The listing builds one solid part. Answer for the finished solid, in the listing's coordinates (mm). Coordinates: 2 decimals unless noted, no trailing zeros. Answer in a Markdown table with one row per item. Add a question column.
```python
from build123d import *

# Parameters (mm, degrees)
BOSS_EXTRUDE1_DEPTH    = 3.175
SKETCH2_R              = 17.4625
CUT_EXTRUDE1_DEPTH     = 435.789559011
F_10_CLEARANCE_HOLE1_D = 5.1054
SKETCH4_R              = 2.794
CUT_EXTRUDE2_DEPTH     = 435.789559011
SKETCH7_R              = 3.048
CUT_EXTRUDE3_DEPTH     = 435.789559011
SKETCH8_R              = 3
CUT_EXTRUDE4_DEPTH     = 435.789559011


with BuildPart() as part:
    # Sketch1 → Boss-Extrude1 (new body)
    with BuildSketch(Plane.XY):
        with BuildLine():
            Line((0, 0), (406.4, 0))
            ThreePointArc((406.4, 0), (431.8, 25.4), (406.4, 50.8))
            Line((406.4, 50.8), (0, 50.8))
            ThreePointArc((0, 50.8), (-25.4, 25.4), (0, 0))
        make_face()
    extrude(amount=BOSS_EXTRUDE1_DEPTH)

    # Sketch2 → Cut-Extrude1 (cut, through all)
    with BuildSketch(Plane.XY.offset(3.175)):
        with Locations((0, 25.4)):
            Circle(SKETCH2_R)
        with Locations((406.4, 25.4)):
            Circle(SKETCH2_R)
    extrude(amount=-CUT_EXTRUDE1_DEPTH, mode=Mode.SUBTRACT)

    # #10 Clearance Hole1 (through all)
    with Locations(Plane(origin=(18.257547563, 35.941, 3.175), x_dir=(1, 0, 0), z_dir=(0, 0, 1))):
        with Locations((0, 0), (0, -21.082), (-18.257547563, -31.623), (-36.515095126, -21.082), (-36.515095126, 0), (-18.257547563, 10.541)):
            Hole(F_10_CLEARANCE_HOLE1_D / 2)

    # Sketch4 → Cut-Extrude2 (cut, through all)
    with BuildSketch(Plane.XY.offset(3.175)):
        with Locations((101.6, 25.4)):
            Circle(SKETCH4_R)
        with Locations((127, 25.4)):
            Circle(SKETCH4_R)
        with Locations((184.272931293, 25.4)):
            Circle(SKETCH4_R)
        with Locations((209.672931293, 25.4)):
            Circle(SKETCH4_R)
    extrude(amount=-CUT_EXTRUDE2_DEPTH, mode=Mode.SUBTRACT)

    # Sketch7 → Cut-Extrude3 (cut, through all)
    with BuildSketch(Plane.XY.offset(3.175)):
        with Locations((306.015176825, 42.672)):
            Circle(SKETCH7_R)
        with Locations((285.695176825, 42.672)):
            Circle(SKETCH7_R)
        with Locations((265.375176825, 42.672)):
            Circle(SKETCH7_R)
    extrude(amount=-CUT_EXTRUDE3_DEPTH, mode=Mode.SUBTRACT)

    # Sketch8 → Cut-Extrude4 (cut, through all)
    with BuildSketch(Plane.XY.offset(3.175)):
        with Locations((323.195176825, 11.543289628)):
            Circle(SKETCH8_R)
        with Locations((323.195176825, 28.543289628)):
            Circle(SKETCH8_R)
        with Locations((248.195176825, 11.543289628)):
            Circle(SKETCH8_R)
        with Locations((248.195176825, 28.543289628)):
            Circle(SKETCH8_R)
    extrude(amount=-CUT_EXTRUDE4_DEPTH, mode=Mode.SUBTRACT)


solid = part.part
```
Q1. A cutting plane is placed at A-A (z = 2.3). State how many separate pieces and enclosed holes the cut face has, then the cut area to 3 significant figures.
Q2. Determine the mould class of faces 1 (the face through (-25.394, 25.959, 1.565)), 2 (the face through (388.954, 26.168, 1.61)), 3 (the face through (200, 26, 3.175)) for opening direction X: +X half, -X half, draft (parallel to the pull), parting line (faces both ways), or undercut.
Q3. Given pin 1 (8 mm diameter, centred on x = 248.2, y = 11.54, fed in from +Z) (3 decimals); pin 2 (5.5 mm diameter, centred on x = 323.2, y = 28.54, fed in from -Z), each flat-ended and moving along its own axis, determine where each tip first touches the part or whether it passes through.
Q4. Straight lines are drawn through the part: line 1 (Y direction, x = 0, z = 1.2); line 2 (X direction, y = 33, z = 1); line 3 (X direction, y = 29, z = 0.35). For each, find the intervals that lie inside material, in ascending order.
Returned:
| question | item | result |
|---|---|---|
| 1 | separate pieces | 1 |
| 1 | enclosed holes | 19 |
| 1 | area | 20,300 mm² |
| 2 | face 1 | -X half |
| 2 | face 2 | undercut |
| 2 | face 3 | draft |
| 3 | pin 1 | stops at z = 3.175 |
| 3 | pin 2 | passes through |
| 4 | line 1 | y = 0 to 1.77, 6.87 to 7.94, 42.86 to 43.93, 49.03 to 50.8 |
| 4 | line 2 | x = -24.24 to -15.72, 15.72 to 390.68, 422.12 to 430.64 |
| 4 | line 3 | x = -25.14 to -17.09, 17.09 to 245.23, 251.16 to 320.23, 326.16 to 389.31, 423.49 to 431.54 |
